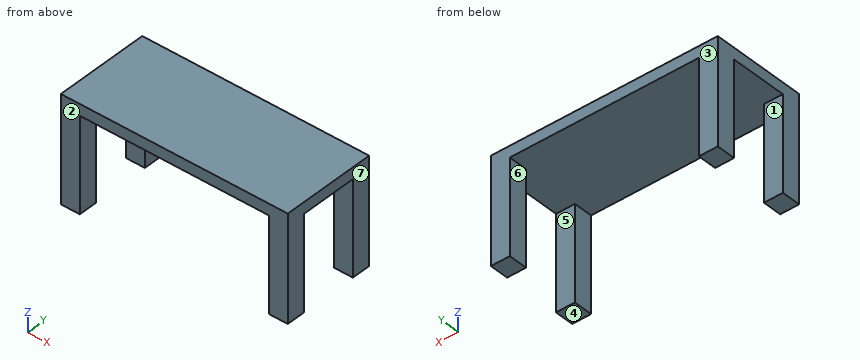
```python
from build123d import *

# Parameters (mm, degrees)
BOSS_EXTRU_1_DEPTH      = 25
ESQUISSE2_W             = 25
ESQUISSE2_H             = 15
ENL_V_MAT_EXTRU_1_DEPTH = 106


with BuildPart() as part:
    # Esquisse1 → Boss.-Extru.1 (new body)
    with BuildSketch(Plane(origin=(0, 0, 0), x_dir=(1, 0, 0), z_dir=(0, 1, 0))):
        Polygon((36.864864865, -13.885135135), (36.864864865, 11.114864865), (41.864864865, 11.114864865), (41.864864865, -16.885135135), (36.864864865, -16.885135135), (-13.135135135, -16.885135135), (-18.135135135, -16.885135135), (-18.135135135, 11.114864865), (-13.135135135, 11.114864865), (-13.135135135, -13.885135135), align=None)
    extrude(amount=BOSS_EXTRU_1_DEPTH)

    # Esquisse2 → Enlèv. mat.-Extru.1 (cut)
    with BuildSketch(Plane(origin=(41.864864865, 0, 0), x_dir=(0, 0, -1), z_dir=(1, 0, 0))):
        with Locations((-1.385135135, 12.5)):
            Rectangle(ESQUISSE2_W, ESQUISSE2_H)
    extrude(amount=-ENL_V_MAT_EXTRU_1_DEPTH, mode=Mode.SUBTRACT)


solid = part.part
```
Could you check a few things on this model? Use its own coordinates, in mm. Face numbers are marked on the shaded views. A direction names the side the tool comes from. Coordinates: 2 decimals unless noted, no trailing zeros. Order: outer loops, then holes, each group sorted by start corner. A loop starts at its lowest first (then second) coordinate and runs counter-clockwise, first axis right, second up. Notation, with made-up numbers: M -21.75,54.5 L -3.75,54.5 A29 cw -3.75,93.5 Z; hole C 51.5,52.25 d10. An arc over 180 degrees is marked long. Use a Markdown table: item, result. Add a question column.
Q1. I want a section at D-D on y = 7.75. List the corners of the cut face in (x, z) for me, then the cut area to 3 significant figures.
Q2. If I drill on L1, parallel to X at y = 22.25, z = 12; L2, parallel to Y at x = 38.5, z = -2.5; L3, parallel to Z at x = 11.5, y = 3.5, over which ranges is the centre line in solid material (lowest first)?
Q3. I want a section at C-C on y = 3.5. List the corners of the cut face in (x, z) for me, then the cut area to 3 significant figures.
Q4. We'd pull the mould along Y, two halves only. Please class the marked faces 1, 2, 3 and 4: pulls with the +Y half, pulls with the -Y half, needs draft (parallel to the pull), parting line crosses it, or undercut.
Q5. Which directions (+Z, -Z, +X, -X, +Y, -Y) give clear straight access to the entire face, cutting with the end or side of a thin tool? Please do the marked faces 5, 6 and 7.
Q6. I want a section at A-A on z = -2.5. List the corners of the cut face in (x, y) for me, then the cut area to 3 significant figures.
Q7. I want a section at B-B on x = 38.5. List the corners of the cut face in (y, z) for me, then the cut area to 3 significant figures.
Q8. I'm going to push flat-ended pins straight in: pin 1 (1 mm diameter, centred on x = 33.5, y = 17.5, fed in from -Z); pin 2 (8 mm diameter, centred on y = 13, z = 0.5, fed in from -X); pin 3 (1.5 mm diameter, centred on x = -15.5, z = -1, fed in from -Y). Where does each tip first touch, or does it pass through?
Checked values:
| question | item | result |
|---|---|---|
| 1 | outline | M -18.14,13.89 L 41.86,13.89 L 41.86,16.89 L -18.14,16.89 Z |
| 1 | area | 180 mm² |
| 2 | L1 | -18.14 to -13.14, 36.86 to 41.86 |
| 2 | L2 | 0 to 5, 20 to 25 |
| 2 | L3 | 13.89 to 16.89 |
| 3 | outline | M -18.14,-11.11 L -13.14,-11.11 L -13.14,13.89 L 36.86,13.89 L 36.86,-11.11 L 41.86,-11.11 L 41.86,16.89 L -18.14,16.89 Z |
| 3 | area | 430 mm² |
| 4 | face 1 | undercut |
| 4 | face 2 | pulls with the -Y half |
| 4 | face 3 | pulls with the +Y half |
| 4 | face 4 | needs draft |
| 5 | face 5 | -Z, +X, -X |
| 5 | face 6 | -Z, +Y, -Y |
| 5 | face 7 | +Z, -Z, +X, +Y, -Y |
| 6 | outline | M -18.14,0 L -13.14,0 L -13.14,5 L -18.14,5 Z; M -18.14,20 L -13.14,20 L -13.14,25 L -18.14,25 Z; M 36.86,0 L 41.86,0 L 41.86,5 L 36.86,5 Z; M 36.86,20 L 41.86,20 L 41.86,25 L 36.86,25 Z |
| 6 | area | 100 mm² |
| 7 | outline | M 0,-11.11 L 5,-11.11 L 5,13.89 L 20,13.89 L 20,-11.11 L 25,-11.11 L 25,16.89 L 0,16.89 Z |
| 7 | area | 325 mm² |
| 8 | pin 1 | z = 13.89 |
| 8 | pin 2 | through |
| 8 | pin 3 | y = 0 |
